The listing builds one solid part. Answer for the finished solid, in the listing's coordinates (mm). A direction names the side the tool comes from. Coordinates: 2 decimals unless noted, no trailing zeros. Order: outer loops, then holes, each group sorted by start corner. A loop starts at its lowest first (then second) coordinate and runs counter-clockwise, first axis right, second up. Notation, with made-up numbers: (54, -18.5) -> (104, -18.5) arc R30 cw to (104, 20.5) -> close; hole circle Ø1 at (-3, 28). An arc over 180 degrees is marked (long way). Return JSON: item names as keys, results as strings.
```python
from build123d import *

# Parameters (mm, degrees)
BOSS_EXTRUDE1_DEPTH = 5
SKETCH2_R           = 1.75
CUT_EXTRUDE1_DEPTH  = 10
SKETCH3_R           = 1.75
CUT_EXTRUDE2_DEPTH  = 10
CUT_EXTRUDE3_DEPTH  = 65
SKETCH5_W           = 54.4
SKETCH5_H           = 38
CUT_EXTRUDE4_DEPTH  = 5
CUT_EXTRUDE5_DEPTH  = 5


with BuildPart() as part:
    # Sketch1 → Boss-Extrude1 (new body)
    with BuildSketch(Plane(origin=(0, 0, 0), x_dir=(1, 0, 0), z_dir=(0, 1, 0))):
        with BuildLine():
            Line((34, -89), (33, -89))
            ThreePointArc((33, -89), (32.292893219, -89.292893219), (32, -90))
            Line((32, -90), (32, -95))
            ThreePointArc((32, -95), (31.707106781, -95.707106781), (31, -96))
            Line((31, -96), (23, -96))
            ThreePointArc((23, -96), (22.292893219, -95.707106781), (22, -95))
            Line((22, -95), (22, -90))
            ThreePointArc((22, -90), (21.707106781, -89.292893219), (21, -89))
            Line((21, -89), (-21, -89))
            ThreePointArc((-21, -89), (-21.707106781, -89.292893219), (-22, -90))
            Line((-22, -90), (-22, -95))
            ThreePointArc((-22, -95), (-22.292893219, -95.707106781), (-23, -96))
            Line((-23, -96), (-31, -96))
            ThreePointArc((-31, -96), (-31.707106781, -95.707106781), (-32, -95))
            Line((-32, -95), (-32, -90))
            ThreePointArc((-32, -90), (-32.292893219, -89.292893219), (-33, -89))
            Line((-33, -89), (-34, -89))
            ThreePointArc((-34, -89), (-34.707106781, -88.707106781), (-35, -88))
            Line((-35, -88), (-35, 88))
            ThreePointArc((-35, 88), (-34.707106781, 88.707106781), (-34, 89))
            Line((-34, 89), (-33, 89))
            ThreePointArc((-33, 89), (-32.292893219, 89.292893219), (-32, 90))
            Line((-32, 90), (-32, 95))
            ThreePointArc((-32, 95), (-31.707106781, 95.707106781), (-31, 96))
            Line((-31, 96), (-23, 96))
            ThreePointArc((-23, 96), (-22.292893219, 95.707106781), (-22, 95))
            Line((-22, 95), (-22, 90))
            ThreePointArc((-22, 90), (-21.707106781, 89.292893219), (-21, 89))
            Line((-21, 89), (21, 89))
            ThreePointArc((21, 89), (21.707106781, 89.292893219), (22, 90))
            Line((22, 90), (22, 95))
            ThreePointArc((22, 95), (22.292893219, 95.707106781), (23, 96))
            Line((23, 96), (31, 96))
            ThreePointArc((31, 96), (31.707106781, 95.707106781), (32, 95))
            Line((32, 95), (32, 90))
            ThreePointArc((32, 90), (32.292893219, 89.292893219), (33, 89))
            Line((33, 89), (34, 89))
            ThreePointArc((34, 89), (34.707106781, 88.707106781), (35, 88))
            Line((35, 88), (35, -88))
            ThreePointArc((35, -88), (34.707106781, -88.707106781), (34, -89))
        make_face()
    extrude(amount=BOSS_EXTRUDE1_DEPTH)

    # Sketch2 → Cut-Extrude1 (cut)
    with BuildSketch(Plane(origin=(0, 5, 0), x_dir=(1, 0, 0), z_dir=(0, 1, 0))):
        with Locations((-20.955, 75)):
            Circle(SKETCH2_R)
        with Locations((-24.13, 8.96)):
            Circle(SKETCH2_R)
        with Locations((20.955, 75)):
            Circle(SKETCH2_R)
        with Locations((24.13, 8.96)):
            Circle(SKETCH2_R)
    extrude(amount=-CUT_EXTRUDE1_DEPTH, mode=Mode.SUBTRACT)

    # Sketch3 → Cut-Extrude2 (cut)
    with BuildSketch(Plane(origin=(0, 5, 0), x_dir=(1, 0, 0), z_dir=(0, 1, 0))):
        with Locations((-31.2, -84)):
            Circle(SKETCH3_R)
        with Locations((31.2, -84)):
            Circle(SKETCH3_R)
        with Locations((31.2, -50.4)):
            Circle(SKETCH3_R)
        with Locations((-31.2, -50.4)):
            Circle(SKETCH3_R)
    extrude(amount=-CUT_EXTRUDE2_DEPTH, mode=Mode.SUBTRACT)

    # Sketch4 → Cut-Extrude3 (cut)
    with BuildSketch(Plane(origin=(0, 5, 0), x_dir=(1, 0, 0), z_dir=(0, 1, 0))):
        with BuildLine():
            Line((-26.2, -84), (26.2, -84))
            ThreePointArc((26.2, -84), (26.907106781, -83.707106781), (27.2, -83))
            Line((27.2, -83), (27.2, -50.4))
            Line((27.2, -50.4), (-27.2, -50.4))
            Line((-27.2, -50.4), (-27.2, -72.4))
            Line((-27.2, -72.4), (-27.2, -83))
            ThreePointArc((-27.2, -83), (-26.907106781, -83.707106781), (-26.2, -84))
        make_face()
    extrude(amount=-CUT_EXTRUDE3_DEPTH, mode=Mode.SUBTRACT)

    # Sketch5 → Cut-Extrude4 (cut)
    with BuildSketch(Plane(origin=(0, 5, 0), x_dir=(1, 0, 0), z_dir=(0, 1, 0))):
        with Locations((0, -31.4)):
            Rectangle(SKETCH5_W, SKETCH5_H)
    extrude(amount=-CUT_EXTRUDE4_DEPTH, mode=Mode.SUBTRACT)

    # Sketch6 → Cut-Extrude5 (cut)
    with BuildSketch(Plane(origin=(0, 5, 0), x_dir=(1, 0, 0), z_dir=(0, 1, 0))):
        with BuildLine():
            Line((26.2, 12.46), (21, 12.46))
            ThreePointArc((21, 12.46), (20.292893219, 12.167106781), (20, 11.46))
            Line((20, 11.46), (20, 6.46))
            ThreePointArc((20, 6.46), (20.292893219, 5.752893219), (21, 5.46))
            Line((21, 5.46), (26.2, 5.46))
            ThreePointArc((26.2, 5.46), (26.907106781, 5.167106781), (27.2, 4.46))
            Line((27.2, 4.46), (27.2, -12.54))
            Line((27.2, -12.54), (16, -12.54))
            Line((16, -12.54), (-20, -12.54))
            Line((-20, -12.54), (-27.2, -12.54))
            Line((-27.2, -12.54), (-27.2, 4.46))
            ThreePointArc((-27.2, 4.46), (-26.907106781, 5.167106781), (-26.2, 5.46))
            Line((-26.2, 5.46), (-21, 5.46))
            ThreePointArc((-21, 5.46), (-20.292893219, 5.752893219), (-20, 6.46))
            Line((-20, 6.46), (-20, 11.46))
            ThreePointArc((-20, 11.46), (-20.292893219, 12.167106781), (-21, 12.46))
            Line((-21, 12.46), (-26.2, 12.46))
            ThreePointArc((-26.2, 12.46), (-26.907106781, 12.752893219), (-27.2, 13.46))
            Line((-27.2, 13.46), (-27.2, 68))
            ThreePointArc((-27.2, 68), (-26.907106781, 68.707106781), (-26.2, 69))
            Line((-26.2, 69), (26.2, 69))
            ThreePointArc((26.2, 69), (26.907106781, 68.707106781), (27.2, 68))
            Line((27.2, 68), (27.2, 13.46))
            ThreePointArc((27.2, 13.46), (26.907106781, 12.752893219), (26.2, 12.46))
        make_face()
    extrude(amount=-CUT_EXTRUDE5_DEPTH, mode=Mode.SUBTRACT)


solid = part.part
```
Item 1: Determine the mould class of faces 6 (the flat face through (32, 2, 92)), 7 (the flat face through (-27, 2, 96)), 8 (the cylindrical face through (-21.33, 2.54, -73.29)) for opening direction X: pulls with the +X half, pulls with the -X half, needs draft (parallel to the pull), parting line crosses it, or undercut.
Answer list:
{"face 6": "pulls with the +X half", "face 7": "needs draft", "face 8": "undercut"}
Item 2: Flat-ended cylindrical pins translate along their axes: pin 1 (2.5 mm diameter, centred on x = -1, y = 3.5, fed in from +Z); pin 2 (1.5 mm diameter, centred on y = 3.5, z = 92.5, fed in from -X); pin 3 (10 mm diameter, centred on x = 17.5, z = 53.5, fed in from -Y). Find the tip coordinate at first contact, or state that the pin passes through.
Answer list:
{"pin 1": "z = 89", "pin 2": "x = -32", "pin 3": "through"}
Item 3: The part is cut by section D-D on y = 3.05. Count the separate pieces of the cut face and the enclosed holes in it, plus the area to 3 significant figures.
Answer list:
{"separate pieces": "1", "enclosed holes": "9", "area": "4,440 mm2"}
Item 4: The part is cut by section B-B on z = 14.5. Determine the outline of the cut face in (x, y), plus the area to 3 significant figures.
Answer list:
{"outline": "(-35, 0) -> (-27.2, 0) -> (-27.2, 5) -> (-35, 5) -> close; (27.2, 0) -> (35, 0) -> (35, 5) -> (27.2, 5) -> close", "area": "78.0 mm2"}
Item 5: The part is cut by section A-A on z = -8.96. Determine the outline of the cut face in (x, y).
Answer list:
{"outline": "(-35, 0) -> (-25.88, 0) -> (-25.88, 5) -> (-35, 5) -> close; (-22.38, 0) -> (-20, 0) -> (-20, 5) -> (-22.38, 5) -> close; (20, 0) -> (22.38, 0) -> (22.38, 5) -> (20, 5) -> close; (25.88, 0) -> (35, 0) -> (35, 5) -> (25.88, 5) -> close"}
Item 6: The part is cut by section C-C on z = -75. Determine the outline of the cut face in (x, y) (3 decimals).
Answer list:
{"outline": "(-35, 0) -> (-22.705, 0) -> (-22.705, 5) -> (-35, 5) -> close; (-19.205, 0) -> (19.205, 0) -> (19.205, 5) -> (-19.205, 5) -> close; (22.705, 0) -> (35, 0) -> (35, 5) -> (22.705, 5) -> close"}
Item 7: Which of the six approach directions +Z, -Z, +X, -X, +Y, -Y give full straight-line access (tool end or side, diameter ignored) to faces 1 (the flat face through (-32, 2, -92)), 2 (the flat face through (27, 2, -96)), 3 (the flat face through (-20, 3, -9)), 4 (the flat face through (22, 2, -92)), 5 (the flat face through (0, 2, 89))?
Answer list:
{"face 1": "-Z, -X, +Y, -Y", "face 2": "-Z, +X, -X, +Y, -Y", "face 3": "+Y, -Y", "face 4": "-Z, +Y, -Y", "face 5": "+Z, +Y, -Y"}
Item 8: Find the intervals of material crossed by probe 1 along X at (y, z) = (3.7, -8.96); probe 2 along X at (y, z) = (3.6, -75) (3 decimals); probe 3 along Z at (x, y) = (31.2, 2.1), in increasing order.
Answer list:
{"probe 1": "-35 to -25.88, -22.38 to -20, 20 to 22.38, 25.88 to 35", "probe 2": "-35 to -22.705, -19.205 to 19.205, 22.705 to 35", "probe 3": "-95.98 to 48.65, 52.15 to 82.25, 85.75 to 95.98"}
